Geometry check sheet. Reference: the model listing, model coordinates, mm. A direction names the side the tool comes from. Coordinates: 2 decimals unless noted, no trailing zeros. Write each loop counter-clockwise with the first axis right and the second up, starting at its lowest first coordinate (ties: lowest second). Pieces come first, ordered by that corner, then holes. Notation, with made-up numbers: M 38.25,-38.75 L 90.25,-38.75 A20 cw 90.25,-24.75 Z; hole C 42.5,-0.5 d11. An arc over 180 degrees is marked long. Put each result on its own line as item: value. Start each with the question number.
1) Scan lines: line 1 along X through (y, z) = (-1, 17.25) (3 decimals); line 2 along X through (y, z) = (6.5, 11); line 3 along Y through (x, z) = (-8, 1.75). Record each from-to range of solid material in increasing order.
2) Set-up check for faces 5 (the flat face through (-53.975, 0, 9)), 6 (the flat face through (-1, 12, 0)): record each of +Z, -Z, +X, -X, +Y, -Y from which the full face is reachable in a straight line by a thin tool's end or side.
3) Gauge pin test, flat end, axial feed: pin 1 (4 mm diameter, centred on x = -64.5, y = 35.5, fed in from -Z). Record the tip position at first contact, or that the pin passes through.
4) Mould release check, pull along X, two halves, no side actions. Record for faces 1 (the flat face through (101.6, -1, 9)), 2 (the flat face through (-1, 50.8, 9)), 3 (the flat face through (-9.144, 0, 9)), 4 (the flat face through (-101.6, -1, 9)): released by +X, released by -X, zero draft, split by the parting line, or undercut.
5) Cross-section at B-B on z = 3. Record the cut outline in (x, y) (3 decimals), plus the area to 3 significant figures.
6) Cross-section at A-A on x = -62.5. Record the cut outline in (y, z) (3 decimals), plus the area to 3 significant figures.
from build123d import *

# Parameters (mm, degrees)
SKETCH1_W           = 203.2
SKETCH1_H           = 101.6
BOSS_EXTRUDE1_DEPTH = 18.25625


with BuildPart() as part:
    # Sketch1 → Boss-Extrude1 (new body)
    with BuildSketch(Plane.XY):
        Rectangle(SKETCH1_W, SKETCH1_H)
        with BuildLine():
            ThreePointArc((-68.534871939, -9.525), (-70.77993597, -10.45493597), (-73.025, -9.525))
            ThreePointArc((-73.025, -9.525), (-73.95493597, -7.27993597), (-73.025, -5.034871939))
            Line((-73.025, -5.034871939), (-73.025, 5.034871939))
            ThreePointArc((-73.025, 5.034871939), (-73.95493597, 7.27993597), (-73.025, 9.525))
            ThreePointArc((-73.025, 9.525), (-70.77993597, 10.45493597), (-68.534871939, 9.525))
            Line((-68.534871939, 9.525), (-58.465128061, 9.525))
            ThreePointArc((-58.465128061, 9.525), (-56.22006403, 10.45493597), (-53.975, 9.525))
            ThreePointArc((-53.975, 9.525), (-53.04506403, 7.27993597), (-53.975, 5.034871939))
            Line((-53.975, 5.034871939), (-53.975, -5.034871939))
            ThreePointArc((-53.975, -5.034871939), (-53.04506403, -7.27993597), (-53.975, -9.525))
            ThreePointArc((-53.975, -9.525), (-56.22006403, -10.45493597), (-58.465128061, -9.525))
            Line((-58.465128061, -9.525), (-68.534871939, -9.525))
        make_face(mode=Mode.SUBTRACT)
        with BuildLine():
            ThreePointArc((-4.653871939, -9.144), (-6.89893597, -10.07393597), (-9.144, -9.144))
            ThreePointArc((-9.144, -9.144), (-10.07393597, -6.89893597), (-9.144, -4.653871939))
            Line((-9.144, -4.653871939), (-9.144, 4.653871939))
            ThreePointArc((-9.144, 4.653871939), (-10.07393597, 6.89893597), (-9.144, 9.144))
            ThreePointArc((-9.144, 9.144), (-6.89893597, 10.07393597), (-4.653871939, 9.144))
            Line((-4.653871939, 9.144), (4.653871939, 9.144))
            ThreePointArc((4.653871939, 9.144), (6.89893597, 10.07393597), (9.144, 9.144))
            ThreePointArc((9.144, 9.144), (10.07393597, 6.89893597), (9.144, 4.653871939))
            Line((9.144, 4.653871939), (9.144, -4.653871939))
            ThreePointArc((9.144, -4.653871939), (10.07393597, -6.89893597), (9.144, -9.144))
            ThreePointArc((9.144, -9.144), (6.89893597, -10.07393597), (4.653871939, -9.144))
            Line((4.653871939, -9.144), (-4.653871939, -9.144))
        make_face(mode=Mode.SUBTRACT)
        with BuildLine():
            ThreePointArc((59.354128061, -8.636), (57.10906403, -9.56593597), (54.864, -8.636))
            ThreePointArc((54.864, -8.636), (53.93406403, -6.39093597), (54.864, -4.145871939))
            Line((54.864, -4.145871939), (54.864, 4.145871939))
            ThreePointArc((54.864, 4.145871939), (53.93406403, 6.39093597), (54.864, 8.636))
            ThreePointArc((54.864, 8.636), (57.10906403, 9.56593597), (59.354128061, 8.636))
            Line((59.354128061, 8.636), (67.645871939, 8.636))
            ThreePointArc((67.645871939, 8.636), (69.89093597, 9.56593597), (72.136, 8.636))
            ThreePointArc((72.136, 8.636), (73.06593597, 6.39093597), (72.136, 4.145871939))
            Line((72.136, 4.145871939), (72.136, -4.145871939))
            ThreePointArc((72.136, -4.145871939), (73.06593597, -6.39093597), (72.136, -8.636))
            ThreePointArc((72.136, -8.636), (69.89093597, -9.56593597), (67.645871939, -8.636))
            Line((67.645871939, -8.636), (59.354128061, -8.636))
        make_face(mode=Mode.SUBTRACT)
    extrude(amount=BOSS_EXTRUDE1_DEPTH)


solid = part.part
Answer key:
1. line 1: x = -101.6 to -73.025, -53.975 to -9.144, 9.144 to 54.864, 72.136 to 101.6
1. line 2: x = -101.6 to -73.86, -53.14 to -10.05, 10.05 to 53.94, 73.06 to 101.6
1. line 3: y = -50.8 to -9.88, 9.88 to 50.8
2. face 5: +Z, -Z
2. face 6: -Z, +X, -X, +Y, -Y
3. pin 1: stops at z = 0
4. face 1: released by +X
4. face 2: zero draft
4. face 3: undercut
4. face 4: released by -X
5. outline: M -101.6,-50.8 L 101.6,-50.8 L 101.6,50.8 L -101.6,50.8 Z; hole M -73.025,-5.035 A3.175 ccw -68.535,-9.525 L -58.465,-9.525 A3.175 ccw -53.975,-5.035 L -53.975,5.035 A3.175 ccw -58.465,9.525 L -68.535,9.525 A3.175 ccw -73.025,5.035 Z; hole M -9.144,-4.654 A3.175 ccw -4.654,-9.144 L 4.654,-9.144 A3.175 ccw 9.144,-4.654 L 9.144,4.654 A3.175 ccw 4.654,9.144 L -4.654,9.144 A3.175 ccw -9.144,4.654 Z; hole M 54.864,-4.146 A3.175 ccw 59.354,-8.636 L 67.646,-8.636 A3.175 ccw 72.136,-4.146 L 72.136,4.146 A3.175 ccw 67.646,8.636 L 59.354,8.636 A3.175 ccw 54.864,4.146 Z
5. area: 19,600 mm²
6. outline: M -50.8,0 L -9.525,0 L -9.525,18.256 L -50.8,18.256 Z; M 9.525,0 L 50.8,0 L 50.8,18.256 L 9.525,18.256 Z
6. area: 1,510 mm²
